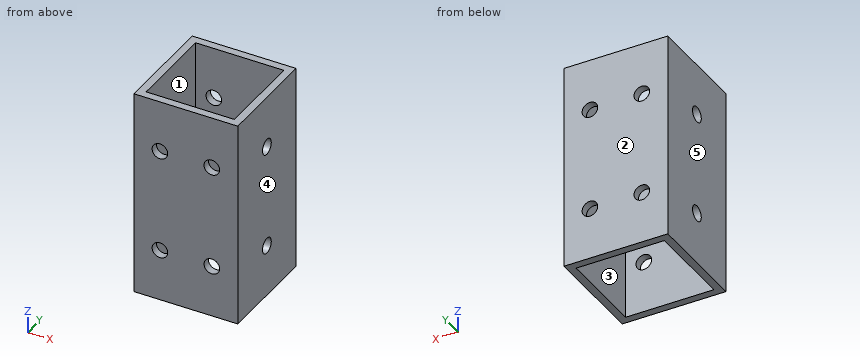
```python
from build123d import *

# Parameters (mm, degrees)
SKETCH_W        = 40
SKETCH_H        = 40
PAD_DEPTH       = 80
SKETCH001_W     = 34
SKETCH001_H     = 34
POCKET_DEPTH    = 80
SKETCH002_R     = 3
POCKET001_DEPTH = 40
SKETCH003_R     = 3
POCKET002_DEPTH = 40


with BuildPart() as part:
    # Sketch → Pad (new body)
    with BuildSketch(Plane.XY):
        with Locations((20, 20)):
            Rectangle(SKETCH_W, SKETCH_H)
    extrude(amount=PAD_DEPTH)

    # Sketch001 (on Face6 of Pad) → Pocket (cut)
    with BuildSketch(Plane.XY.offset(80)):
        with Locations((20, 20)):
            Rectangle(SKETCH001_W, SKETCH001_H)
    extrude(amount=-POCKET_DEPTH, mode=Mode.SUBTRACT)

    # Sketch002 (on Face1 of Pocket) → Pocket001 (cut)
    with BuildSketch(Plane(origin=(0, 40, 0), x_dir=(-1, 0, 0), z_dir=(0, 1, 0))):
        with Locations((-30, 60)):
            Circle(SKETCH002_R)
        with Locations((-10, 60)):
            Circle(SKETCH002_R)
        with Locations((-30, 20)):
            Circle(SKETCH002_R)
        with Locations((-10, 20)):
            Circle(SKETCH002_R)
    extrude(amount=-POCKET001_DEPTH, mode=Mode.SUBTRACT)

    # Sketch003 (on Face5 of Pocket001) → Pocket002 (cut)
    with BuildSketch(Plane.YZ.offset(40)):
        with Locations((20, 60)):
            Circle(SKETCH003_R)
        with Locations((20, 20)):
            Circle(SKETCH003_R)
    extrude(amount=-POCKET002_DEPTH, mode=Mode.SUBTRACT)


solid = part.part
```
CAD build for the part. Positions are in the model's coordinates, mm. Face numbers are marked on the shaded views. A direction names the side the tool comes from. Coordinates: 2 decimals unless noted, no trailing zeros. Order: outer loops, then holes, each group sorted by start corner. A loop starts at its lowest first (then second) coordinate and runs counter-clockwise, first axis right, second up.
(1) Which spindle directions (+Z, -Z, +X, -X, +Y, -Y) get a long thin tool onto all of the face, cutting with end or side? Do the marked faces 1 and 2. Say none if no direction does.
Solution:
face 1: +Z, -Z
face 2: +Z, -Z, +X, -X, +Y
(2) Mould opens along X. For the marked faces 3, 4 and 5 say: released by +X, released by -X, zero draft, split by the parting line, or undercut.
Solution:
face 3: undercut
face 4: released by +X
face 5: released by -X
(3) Saw through at C-C, the plane z = 37.5. Write the cut outline in (x, y).
Solution:
outline: (0, 0) - (40, 0) - (40, 40) - (0, 40) - close; hole (3, 3) - (37, 3) - (37, 37) - (3, 37) - close
(4) Pin check, flat tip, straight feed: pin 1 Ø5.5 at (y, z) = (20, 60) entering from +X. Stop position of the tip, or through.
Solution:
pin 1: passes through
(5) Drill centre lines: L1, parallel to Z at x = 30, y = 38.25; L2, parallel to X at y = 24, z = 22. Where is each one in solid material? Low to high.
Solution:
L1: z = 0 to 17, 23 to 57, 63 to 80
L2: x = 0 to 3, 37 to 40
(6) Saw through at D-D, the plane x = 30. Write the cut outline in (y, z).
Solution:
outline: (0, 0) - (3, 0) - (3, 17) - (0, 17) - close; (0, 23) - (3, 23) - (3, 57) - (0, 57) - close; (0, 63) - (3, 63) - (3, 80) - (0, 80) - close; (37, 0) - (40, 0) - (40, 17) - (37, 17) - close; (37, 23) - (40, 23) - (40, 57) - (37, 57) - close; (37, 63) - (40, 63) - (40, 80) - (37, 80) - close
(7) Saw through at A-A, the plane y = 9. Write the cut outline in (x, z).
Solution:
outline: (0, 0) - (3, 0) - (3, 80) - (0, 80) - close; (37, 0) - (40, 0) - (40, 80) - (37, 80) - close
